Autodesk Inventor part; units mm, degrees
ref_plane "YZ Plane" through (0, 0, 0) normal (1, 0, 0) x (0, 1, 0)
ref_plane "XZ Plane" through (0, 0, 0) normal (0, 1, 0) x (-1, 0, 0)
ref_plane "XY Plane" through (0, 0, 0) normal (0, 0, 1) x (1, 0, 0)
sketch "Sketch1" plane through (0, 0, 0) normal (0, 0, 1) x (1, 0, 0)
  circle A0 centre (0, 0) radius 6
  line L0 (-3, -5.1962) -> (-7.3323, -12.7)
  line L1 (-7.3323, -12.7) -> (7.3323, -12.7)
  line L2 (7.3323, -12.7) -> (3, -5.1962)
  line L3 (-7.5, -22.5) -> (7.5, -22.5)
  line L4 (7.5, -22.5) -> (7.5, -12.7)
  line L5 (7.5, -12.7) -> (-7.5, -12.7)
  line L6 (-7.5, -12.7) -> (-7.5, -22.5)
  line L7 (0, -12.7) -> (0, 0)
  line L8 (-17, -18) -> (17, -18)
  line L9 (17, -18) -> (17, -22.5)
  line L10 (17, -22.5) -> (-17, -22.5)
  line L11 (-17, -22.5) -> (-17, -18)
  point P0 (0, -22.5)
  dimension "d0" = 12
  dimension "d1" = 60
  dimension "d2" = 3
  dimension "d3" = 3
  dimension "d4" = 15
  dimension "d5" = 9.8
  dimension "d7" = 4.5
  dimension "d8" = 34
  dimension "d31" = 22.5
extrude "Extrusion1" add sketch "Sketch1" along normal blind 350
sketch "Sketch2" plane through (0, 0, 350) normal (0, 0, 1) x (1, 0, 0)
  arc A0 (3, -5.1962) -> (-3, -5.1962) centre (0, 0) ccw
  line L0 (3, -5.1962) -> (7.3323, -12.7)
  line L1 (7.3323, -12.7) -> (7.5, -12.7)
  line L2 (7.5, -12.7) -> (7.5, -18)
  line L3 (7.5, -18) -> (17, -18)
  line L4 (17, -18) -> (17, -22.5)
  line L5 (17, -22.5) -> (-17, -22.5)
  line L6 (-17, -22.5) -> (-17, -18)
  line L7 (-17, -18) -> (-7.5, -18)
  line L8 (-7.5, -18) -> (-7.5, -12.7)
  line L9 (-7.5, -12.7) -> (-7.3323, -12.7)
  line L10 (-7.3323, -12.7) -> (-3, -5.1962)
  line L11 (-6, -21.5) -> (6, -21.5)
  line L12 (6, -21.5) -> (6, -22.5)
  line L13 (6, -22.5) -> (-6, -22.5)
  line L14 (-6, -22.5) -> (-6, -21.5)
  point P0 (0, -22.5)
  dimension "d11" = 12
  dimension "d12" = 1
extrude "Extrusion2" cut sketch "Sketch2" against normal through all contours L5 L14 L11 L12
chamfer "Chamfer1" distance 1 angle 45 2 edges at (-6, -21.5, 175) (6, -21.5, 175)
sketch "Sketch3" plane through (-17, -22.5, 0) normal (0, -1, 0) x (1, 0, 0)
  line L0 (23, 0) -> (23, 350) construction
  line L1 (23, 350) -> (34, 350)
  line L2 (34, 350) -> (34, 0)
  line L3 (34, 0) -> (23, 0) construction
  line L4 (11, 350) -> (11, 0) construction
  line L5 (11, 0) -> (0, 0) construction
  line L6 (0, 0) -> (0, 350)
  line L7 (0, 350) -> (11, 350)
  circle A0 centre (4.5, 25) radius 2.55
  circle A1 centre (29.5, 25) radius 2.55
  line L8 (29.5, 25) -> (4.5, 25) construction
  line L9 (17, 25) -> (17, 0) construction
  dimension "d18" = 25
  dimension "d19" = 5.1
  dimension "d20" = 5.1
  dimension "d21" = 25
extrude "Extrusion3" cut sketch "Sketch3" against normal through all
pattern_linear "Rectangular Pattern1" count 4 spacing 100 along (0, 0, 1) of "Extrusion3"
sketch "Sketch4" plane through (0, 0, 0) normal (0, 0, -1) x (-1, 0, 0)
  line L0 (-5, -21.5) -> (-6, -22.5)
  line L1 (-5, -21.5) -> (5, -21.5)
  line L2 (6, -22.5) -> (5, -21.5)
  line L3 (17, -22.5) -> (6, -22.5)
  line L4 (17, -18) -> (17, -22.5)
  line L5 (7.5, -18) -> (17, -18)
  line L6 (7.5, -12.7) -> (7.5, -18)
  line L7 (7.3323, -12.7) -> (7.5, -12.7)
  line L8 (3, -5.1962) -> (7.3323, -12.7)
  arc A0 (3, -5.1962) -> (-3, -5.1962) centre (0, 0) ccw
  line L9 (-7.3323, -12.7) -> (-3, -5.1962)
  line L10 (-7.5, -12.7) -> (-7.3323, -12.7)
  line L11 (-7.5, -18) -> (-7.5, -12.7)
  line L12 (-17, -18) -> (-7.5, -18)
  line L13 (-17, -22.5) -> (-17, -18)
  line L14 (-6, -22.5) -> (-17, -22.5)
  circle A1 centre (0, 0) radius 6
extrude "Extrusion4" cut sketch "Sketch4" against normal blind 0.5 contours A0 A1
sketch "Sketch5" plane through (0, 0, 350) normal (0, 0, 1) x (1, 0, 0)
  line L0 (6, -22.5) -> (17, -22.5)
  line L1 (17, -22.5) -> (17, -18)
  line L2 (17, -18) -> (7.5, -18)
  line L3 (7.5, -18) -> (7.5, -12.7)
  line L4 (7.5, -12.7) -> (7.3323, -12.7)
  line L5 (7.3323, -12.7) -> (3, -5.1962)
  arc A0 (3, -5.1962) -> (-3, -5.1962) centre (0, 0) ccw
  line L6 (-3, -5.1962) -> (-7.3323, -12.7)
  line L7 (-7.3323, -12.7) -> (-7.5, -12.7)
  line L8 (-7.5, -12.7) -> (-7.5, -18)
  line L9 (-7.5, -18) -> (-17, -18)
  line L10 (-17, -18) -> (-17, -22.5)
  line L11 (-17, -22.5) -> (-6, -22.5)
  line L12 (-5, -21.5) -> (-6, -22.5)
  line L13 (-5, -21.5) -> (5, -21.5)
  line L14 (6, -22.5) -> (5, -21.5)
  circle A1 centre (0, 0) radius 6
extrude "Extrusion5" cut sketch "Sketch5" against normal blind 0.5 contours A1 A0
properties part number "sbr12_350mm"
Input: part model. Units: mm. Frame: model coordinates. A direction names the side the tool comes from. Coordinates: 2 decimals unless noted, no trailing zeros. Write each loop counter-clockwise with the first axis right and the second up, starting at its lowest first coordinate (ties: lowest second). Pieces come first, ordered by that corner, then holes. Notation, with made-up numbers: M 41.5,19 L 60.5,19 A13 cw 60.5,41 Z; hole C 1.5,-23 d4. An arc over 180 degrees is marked long. Answer as a JSON object with one key per item and string values. Group by question number.
(1) Mould query, pull axis Y, two halves, no side actions, for faces 1 (the face through (0, 6, 173)), 2 (the face through (0, 0, 349.5)), 3 (the face through (0, -21.5, 177)), 4 (the face through (-12, -18, 173)). Classes: pulls with the +Y half, pulls with the -Y half, needs draft (parallel to the pull), parting line crosses it, or undercut.
(2) Ray query, line 1 along Z through (x, y) = (12.5, -20.5); line 2 along X through (y, z) = (-19, 325); line 3 along Z through (x, y) = (1.5, -1.75). Return the intervals inside material, ascending. Write a range as [from, to].
(3) Section C-C on y = 0. Output: boundary loops of the cut face in (x, z).
(4) Set-up query: faces 5 (the face through (12, -18, 173)), 6 (the face through (-5.14, -8.9, 172.55)), 7 (the face through (5.196, -9.001, 172.55)), 8 (the face through (-7.5, -15, 173)). Return all of +Z, -Z, +X, -X, +Y, -Y with unobstructed straight access to the full face (end or side cutting, diameter ignored); none if empty.
(5) Section A-A on x = 0. Output: boundary loops of the cut face in (y, z).
(6) Contact query for flat-ended pins moving along their axis: P1, Ø1, axis at y = 1, z = 139.5, coming from the -X side; P2, Ø3.5, axis at x = 1, y = 1.5, coming from the +Z side; P3, Ø3.5, axis at x = 0, y = -2.5, coming from the -Z side; P4, Ø4.5, axis at x = 12.5, z = 25, coming from the -Y side. Output: stop coordinate, or through.
Result set:
{
 "1": {"face 1": "undercut", "face 2": "needs draft", "face 3": "pulls with the -Y half", "face 4": "pulls with the +Y half"},
 "2": {"line 1": "z = [0, 22.45], [27.55, 122.45], [127.55, 222.45], [227.55, 322.45], [327.55, 350]", "line 2": "x = [-17, -15.05], [-9.95, 9.95], [15.05, 17]", "line 3": "z = [0.5, 349.5]"},
 "3": {"outline": "M -6,0.5 L 6,0.5 L 6,349.5 L -6,349.5 Z"},
 "4": {"face 5": "+Z, -Z, +X, +Y", "face 6": "+Z, -Z, -X", "face 7": "+Z, -Z, +X", "face 8": "+Z, -Z, -X, +Y"},
 "5": {"outline": "M -21.5,0 L -6,0 L -6,0.5 L 6,0.5 L 6,349.5 L -6,349.5 L -6,350 L -21.5,350 Z"},
 "6": {"P1": "stops at x = -5.98", "P2": "stops at z = 349.5", "P3": "stops at z = 0.5", "P4": "passes through"}
}
